Part model, mm, in its own coordinate system. Face numbers are marked on the shaded views. Give positions to 0.01 mm unless a question says otherwise; leave off trailing zeros. Order: outer loops, then holes, each group sorted by start corner. A loop starts at its lowest first (then second) coordinate and runs counter-clockwise, first axis right, second up. Notation, with made-up numbers: M -13,84 L 8,84 A27 ccw 8,115 Z; hole C 30.25,-33.75 d1. An arc over 180 degrees is marked long. Answer as a JSON object with one key per item and string values.
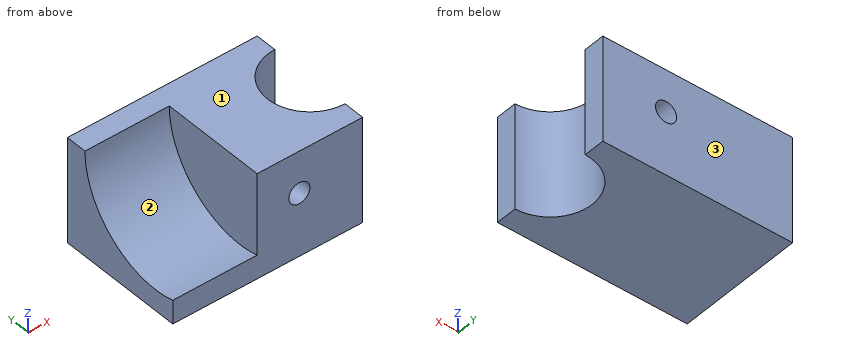
from build123d import *

# Parameters (mm, degrees)
F0_W     = 57.15
F0_H     = 38.1
F1_DEPTH = 31.75
F3_DEPTH = 31.75
F4_R     = 3.175
F5_DEPTH = 37.846
F6_DEPTH = 38.1
F7_R     = 25.4
F8_DEPTH = 25.4


with BuildPart() as f1:
    # F0 (on Top) → F1 (new body)
    with BuildSketch(Plane.XY):
        with Locations((42.536962, -12.618525)):
            Rectangle(F0_W, F0_H)
    extrude(amount=F1_DEPTH)

    # F2 (on face) → F3 (cut)
    with BuildSketch(Plane.XY.offset(31.75)):
        with BuildLine():
            ThreePointArc((71.111962, -25.318525), (80.092218, -21.598781), (83.811962, -12.618525))
            ThreePointArc((83.811962, -12.618525), (80.092218, -3.638269), (71.111962, 0.081475))
            Line((71.111962, 0.081475), (71.111962, -25.318525))
        make_face()
        with BuildLine():
            Line((71.111962, -25.318525), (71.111962, 0.081475))
            ThreePointArc((71.111962, 0.081475), (58.411962, -12.618525), (71.111962, -25.318525))
        make_face()
    extrude(amount=-F3_DEPTH, mode=Mode.SUBTRACT)

    # F4 (on face) → F5 (cut)
    with BuildSketch(Plane.XZ.offset(31.668525)):
        with Locations((52.061962, 19.05)):
            Circle(F4_R)
    extrude(amount=-F5_DEPTH, mode=Mode.SUBTRACT)

    # F4 (on face) → F6 (cut)
    with BuildSketch(Plane.XZ.offset(31.668525)):
        with Locations((52.061962, 19.05)):
            Circle(F4_R)
    extrude(amount=-F6_DEPTH, mode=Mode.SUBTRACT)

    # F7 (on face) → F8 (cut)
    with BuildSketch(Plane(origin=(13.961962, 0, 0), x_dir=(0, -1, 0), z_dir=(-1, 0, 0))):
        with Locations((25.318525, 31.75)):
            Circle(F7_R)
    extrude(amount=-F8_DEPTH, mode=Mode.SUBTRACT)


solid = f1.part
1. Cut at A-A on y = 2.5. Give the cut face in (x, z) (3 decimals).
Worked answers:
{"outline": "M 13.962,0 L 71.112,0 L 71.112,31.75 L 13.962,31.75 Z; hole C 52.062,19.05 d6.35"}
2. Pin check, flat tips, straight feed: P1, Ø10, axis at x = 21, z = 20.5, coming from the -Y side; P2, Ø2, axis at x = 34, y = -15.5, coming from the +Z side; P3, Ø5, axis at x = 54, y = -2.5, coming from the -Z side; P4, Ø3, axis at y = -11.5, z = 4.5, coming from the +X side. Stop position of each tip, or through.
Worked answers:
{"P1": "stops at y = -5.8", "P2": "stops at z = 8.77", "P3": "stops at z = 0", "P4": "stops at x = 58.68"}
3. Cut at D-D on x = 67.5. Give the cut face in (y, z), plus the area to 3 significant figures.
Worked answers:
{"outline": "M -31.67,0 L -24.79,0 L -24.79,31.75 L -31.67,31.75 Z; M -0.44,0 L 6.43,0 L 6.43,31.75 L -0.44,31.75 Z", "area": "437 mm^2"}
4. Probe line 1 along X through (y, z) = (-25.5, 25.5); line 2 along X through (y, z) = (-17.5, 20); line 3 along Z through (x, y) = (53, -15). List the from-to ranges inside material, lowest first.
Worked answers:
{"line 1": "x = 39.36 to 71.11", "line 2": "x = 39.36 to 49.03, 55.09 to 59.39", "line 3": "z = 0 to 16.02, 22.08 to 31.75"}
5. Two-plate mould, pull along Y, no slides. Class the marked faces 1, 2 and 3: +Y half, -Y half, draft (parallel to the pull), parting line (faces both ways), or undercut.
Worked answers:
{"face 1": "draft", "face 2": "undercut", "face 3": "+Y half"}
6. Cut at B-B on z = 5. Give the cut face in (x, y).
Worked answers:
{"outline": "M 13.96,-31.67 L 71.11,-31.67 L 71.11,-25.32 A12.7 cw 71.11,0.08 L 71.11,6.43 L 13.96,6.43 Z"}
7. Cut at C-C on z = 19.05. Give the cut face in (x, y), plus the area to 3 significant figures.
Worked answers:
{"outline": "M 13.96,-3.32 L 39.36,-3.32 L 39.36,-31.67 L 48.89,-31.67 L 48.89,6.43 L 13.96,6.43 Z; M 55.24,-31.67 L 71.11,-31.67 L 71.11,-25.32 A12.7 cw 71.11,0.08 L 71.11,6.43 L 55.24,6.43 Z", "area": "962 mm^2"}
